Study the drawing (mm; zero at the part's minimum x, y, z) and answer. A direction names the side the tool comes from. Give positions to 0.01 mm unless a question says otherwise; leave off trailing zeros. Order: outer loops, then holes, each group sorted by start corner. A loop starts at its lowest first (then second) coordinate and runs counter-clockwise, first axis right, second up. Notation, with made-up numbers: (76.25, 3) -> (128.25, 3) arc R20 cw to (128.25, 42) -> close; hole circle Ø7 at (0, 71). An arc over 180 degrees is marked (long way). Answer as CSV lines item,"result". Start each with the question number.
1. For a pull along Z with two mould halves and no side action, classify the marked faces 1, 2 and 3 as released by +Z, released by -Z, zero draft, split by the parting line, or undercut.
2. Find the intervals of material crossed by L1, parallel to X at y = 4, z = 15; L2, parallel to X at y = 1.65, z = 5; L3, parallel to Z at x = 15, y = 4.35, in increasing order.
3. For the marked faces 4 and 5, determine the directions among +Z, -Z, +X, -X, +Y, -Y from which every point of the face is accessible in a straight line to the end or side of a thin tool.
4. A cutting plane is placed at C-C (x = 5). Give the vertices of the cut face in (y, z).
5. A cutting plane is placed at B-B (z = 14). Give the vertices of the cut face in (x, y).
6. Flat-ended cylindrical pins translate along their axes: pin 1 (1.9 mm diameter, centred on x = 25, z = 15, fed in from -Y); pin 2 (2 mm diameter, centred on y = 2, z = 10.5, fed in from +X); pin 3 (2 mm diameter, centred on y = 4.5, z = 9.5, fed in from -X); pin 4 (1 mm diameter, centred on y = 1.5, z = 8.5, fed in from +X). Find the tip coordinate at first contact, or state that the pin passes through.
7. A cutting plane is placed at D-D (z = 5). Give the vertices of the cut face in (x, y), then the cut area to 3 significant figures.
8. A cutting plane is placed at A-A (x = 15). Give the vertices of the cut face in (y, z).
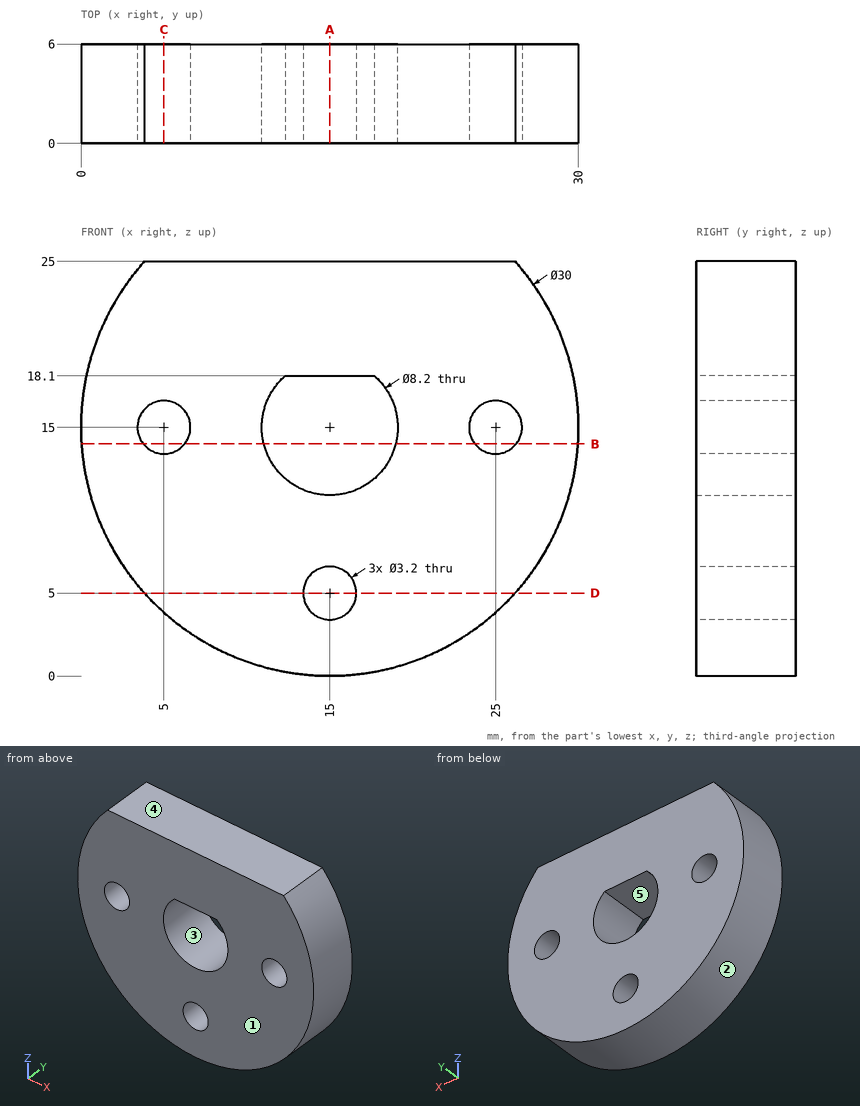
Answer sheet:
1,face 1,"zero draft"
1,face 2,"split by the parting line"
1,face 3,"undercut"
2,L1,"x = 0 to 3.4, 6.6 to 10.9, 19.1 to 23.4, 26.6 to 30"
2,L2,"x = 3.82 to 13.4, 16.6 to 26.18"
2,L3,"z = 0 to 3.4, 6.6 to 10.9, 18.1 to 25"
3,face 4,"+Z, +X, -X, +Y, -Y"
3,face 5,"+Y, -Y"
4,outline,"(0, 3.82) -> (6, 3.82) -> (6, 13.4) -> (0, 13.4) -> close; (0, 16.6) -> (6, 16.6) -> (6, 25) -> (0, 25) -> close"
5,outline,"(0.03, 0) -> (3.75, 0) -> (3.75, 6) -> (0.03, 6) -> close; (6.25, 0) -> (11.02, 0) -> (11.02, 6) -> (6.25, 6) -> close; (18.98, 0) -> (23.75, 0) -> (23.75, 6) -> (18.98, 6) -> close; (26.25, 0) -> (29.97, 0) -> (29.97, 6) -> (26.25, 6) -> close"
6,pin 1,"passes through"
6,pin 2,"stops at x = 29.59"
6,pin 3,"stops at x = 0.69"
6,pin 4,"stops at x = 28.75"
7,outline,"(3.82, 0) -> (13.4, 0) -> (13.4, 6) -> (3.82, 6) -> close; (16.6, 0) -> (26.18, 0) -> (26.18, 6) -> (16.6, 6) -> close"
7,area,"115 mm^2"
8,outline,"(0, 0) -> (6, 0) -> (6, 3.4) -> (0, 3.4) -> close; (0, 6.6) -> (6, 6.6) -> (6, 10.9) -> (0, 10.9) -> close; (0, 18.1) -> (6, 18.1) -> (6, 25) -> (0, 25) -> close"
